from build123d import *

# Parameters (mm, degrees)
F0_W     = 76.2
F0_H     = 25.4
F1_DEPTH = 25.4
F2_W     = 25.4508
F2_H     = 12.7254
F3_DEPTH = 25.4
F4_W     = 25.4508
F4_H     = 12.7254
F5_DEPTH = 25.654
F6_DEPTH = 12.304268


with BuildPart() as f1:
    # F0 (on Top) → F1 (new body)
    with BuildSketch(Plane.XY):
        with Locations((38.1, 12.7)):
            Rectangle(F0_W, F0_H)
    extrude(amount=F1_DEPTH)

    # F2 (on Front) → F3 (cut)
    with BuildSketch(Plane.XZ):
        with Locations((38.1, 19.458432)):
            Rectangle(F2_W, F2_H)
    extrude(amount=-F3_DEPTH, mode=Mode.SUBTRACT)

    # F4 (on Top) → F5 (cut)
    with BuildSketch(Plane.XY):
        with Locations((25.3746, 6.3627)):
            Rectangle(F4_W, F4_H)
    extrude(amount=F5_DEPTH, mode=Mode.SUBTRACT)

    # F3_face (on face) → F6 (join, through all)
    with BuildSketch(Plane(origin=(40.22656, 14.81807, 13.095732), x_dir=(1, 0, 0), z_dir=(0, 0, 1))):
        Polygon((-14.85196, -2.09267), (-2.12656, -2.09267), (-2.12656, -14.81807), (10.59884, -14.81807), (10.59884, 10.58193), (-14.85196, 10.58193), align=None)
    extrude(amount=F6_DEPTH)


solid = f1.part
Design review of the part built by this model. Coordinates are the model's own, in mm. A direction names the side the tool comes from. Give positions to 0.01 mm unless a question says otherwise; leave off trailing zeros. Loops run counter-clockwise (first coordinate to the right, second up) from the corner with the lowest first, then second, coordinate; pieces in that order, holes last. Notation, with made-up numbers: (-39.5, -34) -> (-27.5, -34) arc R22 ccw to (-27.5, -17) -> close; hole circle Ø11 at (29.25, 59.5). An arc over 180 degrees is marked (long way). One line per question, with ' | ' between items. Start each with the question number.
(1) Draft analysis for pull direction X (two halves, no side actions). For faces 1 (the face through (76.2, 13, 13)), 2 (the face through (38.1, 6, 13)), 3 (the face through (25, 12.725, 13)), 4 (the face through (6, 0, 13)), state which applies: +X half, -X half, draft (parallel to the pull), parting line (faces both ways), or undercut.
(2) For faces 5 (the face through (12.649, 6, 13)), 6 (the face through (38, 13, 25.4)), list the 3-axis set-ups (+Z, -Z, +X, -X, +Y, -Y) from which the entire face can be reached by the end or side of a thin tool; tool diameter is ignored.
(3) For line 1 (X direction, y = 7.25, z = 2); line 2 (Y direction, x = 32.5, z = 2), list the stretches that pass through material, from the lowest coordinate up.
(4) We need section B-B (z = 5.75). State the section outline as (x, y) points.
(5) Insertion check: P1, Ø7.5, axis at x = 31, z = 9, coming from the -Y side. The pin has a flat end and moves straight along its axis. Give the tip position at first contact, or say it passes through.
(6) We need section C-C (x = 13.5). State the section outline as (y, z) points.
(7) We need section A-A (y = 6.25). State the section outline as (x, z) points, and give its area (3 significant figures).
The answers:
1) face 1: +X half | face 2: undercut | face 3: undercut | face 4: draft
2) face 5: +Z, -Z, -Y | face 6: +Z, +X, -X, +Y, -Y
3) line 1: x = 0 to 12.65, 38.1 to 76.2 | line 2: y = 12.73 to 25.4
4) outline: (0, 0) -> (12.65, 0) -> (12.65, 12.73) -> (38.1, 12.73) -> (38.1, 0) -> (76.2, 0) -> (76.2, 25.4) -> (0, 25.4) -> close
5) P1: stops at y = 12.73
6) outline: (12.73, 0) -> (25.4, 0) -> (25.4, 25.4) -> (12.73, 25.4) -> close
7) outline: (0, 0) -> (12.65, 0) -> (12.65, 25.4) -> (0, 25.4) -> close; (38.1, 0) -> (76.2, 0) -> (76.2, 25.4) -> (38.1, 25.4) -> close | area: 1,290 mm^2
